Design review of the part built by this model. Coordinates are the model's own, in mm. Face numbers are marked on the shaded views. A direction names the side the tool comes from. Coordinates: 2 decimals unless noted, no trailing zeros. Loops run counter-clockwise (first coordinate to the right, second up) from the corner with the lowest first, then second, coordinate; pieces in that order, holes last. Notation, with made-up numbers: (-12, -32) -> (-4, -32) arc R28 ccw to (-4, -4) -> close; hole circle Ø8 at (61, -15). An arc over 180 degrees is marked (long way). Answer in a Markdown table with one row per item.
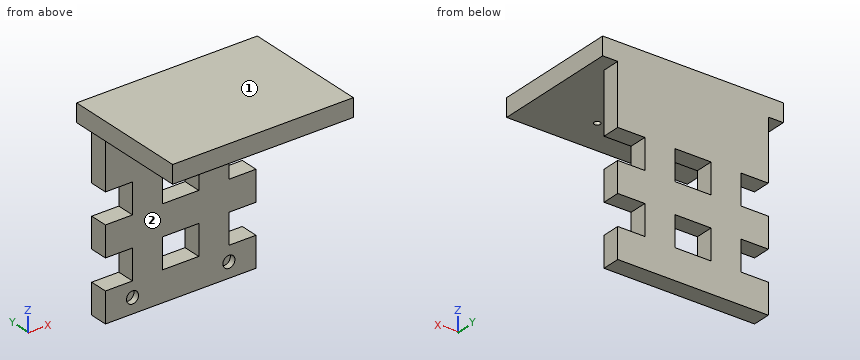
```python
from build123d import *

# Parameters (mm, degrees)
SKETCH1_W           = 300
SKETCH1_H           = 380
BOSS_EXTRUDE1_DEPTH = 30
SKETCH3_W           = 250
SKETCH3_H           = 30
BOSS_EXTRUDE2_DEPTH = 100
BOSS_EXTRUDE3_START = 150
SKETCH3_2_W         = 250
SKETCH3_2_H         = 30
BOSS_EXTRUDE3_DEPTH = 50
BOSS_EXTRUDE4_START = 250
SKETCH3_3_W         = 250
SKETCH3_3_H         = 30
BOSS_EXTRUDE4_DEPTH = 50
SKETCH4_W           = 50
SKETCH4_H           = 30
BOSS_EXTRUDE5_DEPTH = 50
BOSS_EXTRUDE6_START = -50
SKETCH4_2_W         = 50
SKETCH4_2_H         = 30
BOSS_EXTRUDE6_DEPTH = 50
SKETCH5_R           = 10
CUT_EXTRUDE1_DEPTH  = 10
SKETCH6_R           = 5
CUT_EXTRUDE2_DEPTH  = 10
SKETCH7_W           = 300
SKETCH7_H           = 170
CUT_EXTRUDE3_DEPTH  = 30


with BuildPart() as part:
    # Sketch1 → Boss-Extrude1 (new body)
    with BuildSketch(Plane.XY):
        Rectangle(SKETCH1_W, SKETCH1_H)
    extrude(amount=BOSS_EXTRUDE1_DEPTH)

    # Sketch3 → Boss-Extrude2 (add)
    with BuildSketch(Plane(origin=(0, 0, 0), x_dir=(-1, 0, 0), z_dir=(0, 0, -1))):
        with Locations((0, 175)):
            Rectangle(SKETCH3_W, SKETCH3_H)
    extrude(amount=BOSS_EXTRUDE2_DEPTH)



with BuildPart() as body_2:
    # Sketch3_2 → Boss-Extrude3 (new body)
    with BuildSketch(Plane(origin=(0, 0, 0), x_dir=(-1, 0, 0), z_dir=(0, 0, -1)).offset(BOSS_EXTRUDE3_START)):
        with Locations((0, 175)):
            Rectangle(SKETCH3_2_W, SKETCH3_2_H)
    extrude(amount=BOSS_EXTRUDE3_DEPTH)


with BuildPart() as body_3:
    # Sketch3_3 → Boss-Extrude4 (new body)
    with BuildSketch(Plane(origin=(0, 0, 0), x_dir=(-1, 0, 0), z_dir=(0, 0, -1)).offset(BOSS_EXTRUDE4_START)):
        with Locations((0, 175)):
            Rectangle(SKETCH3_3_W, SKETCH3_3_H)
    extrude(amount=BOSS_EXTRUDE4_DEPTH)


with BuildPart() as part_1:
    add(part.part)

    add(body_2.part)  # Boss-Extrude5 merges body 2
    # Sketch4 → Boss-Extrude5 (add)
    with BuildSketch(Plane.XY.offset(-150)):
        with Locations((-55, 175)):
            Rectangle(SKETCH4_W, SKETCH4_H)
        with Locations((55, 175)):
            Rectangle(SKETCH4_W, SKETCH4_H)
    extrude(amount=BOSS_EXTRUDE5_DEPTH)


    add(body_3.part)  # Boss-Extrude6 merges body 3
    # Sketch4_2 → Boss-Extrude6 (add)
    with BuildSketch(Plane.XY.offset(-150).offset(BOSS_EXTRUDE6_START)):
        with Locations((-55, 175)):
            Rectangle(SKETCH4_2_W, SKETCH4_2_H)
        with Locations((55, 175)):
            Rectangle(SKETCH4_2_W, SKETCH4_2_H)
    extrude(amount=-BOSS_EXTRUDE6_DEPTH)

    # Sketch5 → Cut-Extrude1 (cut)
    with BuildSketch(Plane.XZ.offset(-160)):
        with Locations((-80, -275)):
            Circle(SKETCH5_R)
        with Locations((80, -275)):
            Circle(SKETCH5_R)
        with Locations((0, -75)):
            Circle(SKETCH5_R)
    extrude(amount=-CUT_EXTRUDE1_DEPTH, mode=Mode.SUBTRACT)

    # Sketch6 → Cut-Extrude2 (cut)
    with BuildSketch(Plane(origin=(0, 0, 0), x_dir=(-1, 0, 0), z_dir=(0, 0, -1))):
        with Locations((-45, 40)):
            Circle(SKETCH6_R)
        with Locations((45, 40)):
            Circle(SKETCH6_R)
    extrude(amount=-CUT_EXTRUDE2_DEPTH, mode=Mode.SUBTRACT)

    # Sketch7 → Cut-Extrude3 (cut)
    with BuildSketch(Plane(origin=(0, 0, 0), x_dir=(-1, 0, 0), z_dir=(0, 0, -1))):
        with Locations((0, -105)):
            Rectangle(SKETCH7_W, SKETCH7_H)
    extrude(amount=-CUT_EXTRUDE3_DEPTH, mode=Mode.SUBTRACT)


solid = part_1.part
```
(1) Take a section at A-A on x = -23. Give the boundary of the cut face in (y, z).
Evaluation:
| item | result |
|---|---|
| outline | (-20, 0) -> (160, 0) -> (160, -100) -> (190, -100) -> (190, 30) -> (-20, 30) -> close; (160, -300) -> (190, -300) -> (190, -250) -> (160, -250) -> close; (160, -200) -> (190, -200) -> (190, -150) -> (160, -150) -> close |
(2) Take a section at B-B on z = -208. Give the boundary of the cut face in (x, y), and give its area (3 significant figures).
Evaluation:
| item | result |
|---|---|
| outline | (-80, 160) -> (-30, 160) -> (-30, 190) -> (-80, 190) -> close; (30, 160) -> (80, 160) -> (80, 190) -> (30, 190) -> close |
| area | 3,000 mm² |
(3) For pin 1 (10 mm diameter, centred on x = 76.5, z = -271.5, fed in from -Y); pin 2 (16 mm diameter, centred on x = -84, z = -276.5, fed in from -Y); pin 3 (2 mm diameter, centred on x = 18, y = 39, fed in from -Z), all flat-tipped, find the tip position at first contact; note any pin that passes through.
Evaluation:
| item | result |
|---|---|
| pin 1 | stops at y = 170 |
| pin 2 | stops at y = 160 |
| pin 3 | stops at z = 0 |
(4) To check wall thickness, follow probe 1 along Z at (x, y) = (0, 167); probe 2 along Z at (x, y) = (85.5, 181); probe 3 along Y at (x, z) = (-45, 4.5). State the ranges of each line that lie inside material, in increasing order.
Evaluation:
| item | result |
|---|---|
| probe 1 | z = -300 to -250, -200 to -150, -100 to -85, -65 to 30 |
| probe 2 | z = -300 to -250, -200 to -150, -100 to 30 |
| probe 3 | y = -20 to 35, 45 to 190 |
(5) Take a section at D-D on x = 45. Give the boundary of the cut face in (y, z).
Evaluation:
| item | result |
|---|---|
| outline | (-20, 0) -> (35, 0) -> (35, 10) -> (45, 10) -> (45, 0) -> (160, 0) -> (160, -300) -> (190, -300) -> (190, 30) -> (-20, 30) -> close |
(6) Tool access review of the marked faces 1 and 2: name each direction out of +Z, -Z, +X, -X, +Y, -Y from which nothing blocks a thin tool from reaching the whole face with its end or side.
Evaluation:
| item | result |
|---|---|
| face 1 | +Z, +X, -X, +Y, -Y |
| face 2 | -Z, +X, -X, -Y |
(7) Take a section at C-C on y = 40. Give the boundary of the cut face in (x, z).
Evaluation:
| item | result |
|---|---|
| outline | (-150, 0) -> (-50, 0) -> (-50, 10) -> (-40, 10) -> (-40, 0) -> (40, 0) -> (40, 10) -> (50, 10) -> (50, 0) -> (150, 0) -> (150, 30) -> (-150, 30) -> close |
